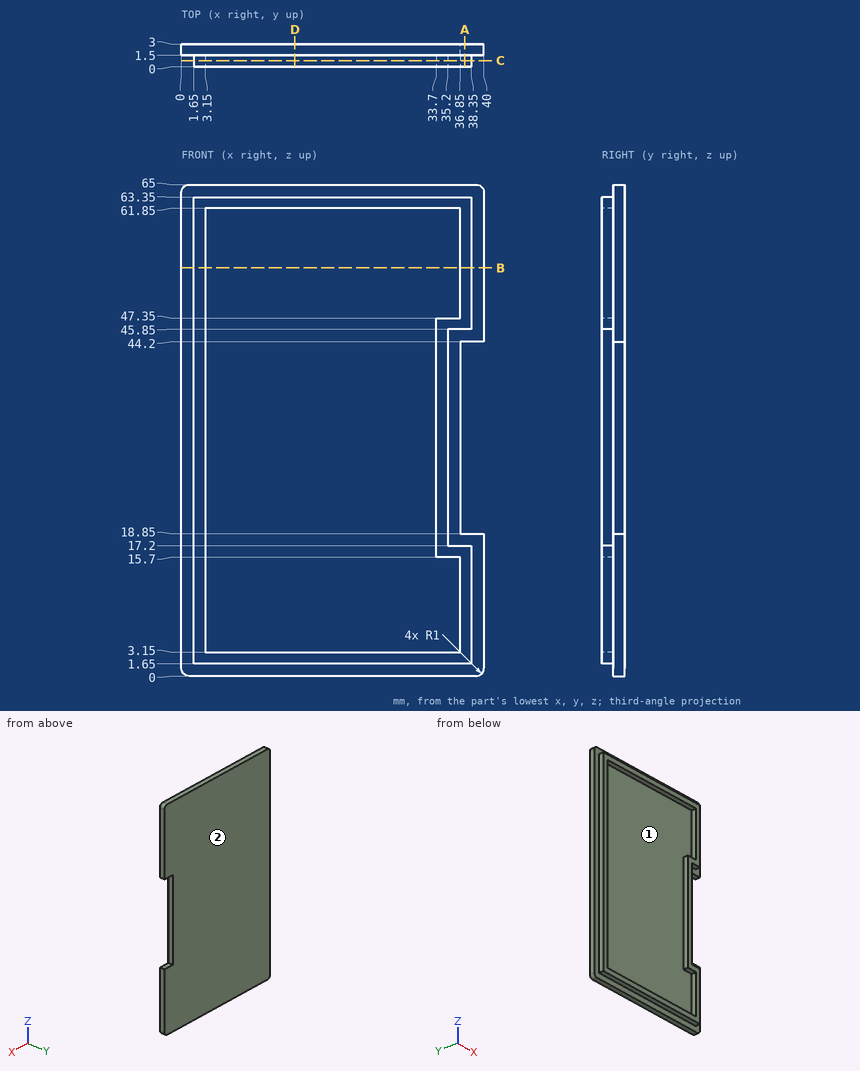
The drawing under review shows one solid part. Ordinate dimensions are in mm from its lowest x, y, z. Round coordinates to 2 decimals unless told otherwise and drop trailing zeros. Write each loop counter-clockwise with the first axis right and the second up, starting at its lowest first coordinate (ties: lowest second). Pieces come first, ordered by that corner, then holes. Notation, with made-up numbers: (33, -22) - (72, -22) arc R20 cw to (72, -12) - close; hole circle Ø10 at (-30, 8). An arc over 180 degrees is marked (long way). Put each result on its own line as item: value.
Q1. We need section D-D (x = 15). Give the boundary of the cut face in (y, z), and give its area (3 significant figures).
Solved:
outline: (0, 1.65) - (1.5, 1.65) - (1.5, 0) - (3, 0) - (3, 65) - (1.5, 65) - (1.5, 63.35) - (0, 63.35) - (0, 61.85) - (1.5, 61.85) - (1.5, 3.15) - (0, 3.15) - close
area: 102 mm2
Q2. We need section B-B (z = 54). Give the boundary of the cut face in (x, y).
Solved:
outline: (0, 1.5) - (1.65, 1.5) - (1.65, 0) - (3.15, 0) - (3.15, 1.5) - (36.85, 1.5) - (36.85, 0) - (38.35, 0) - (38.35, 1.5) - (40, 1.5) - (40, 3) - (0, 3) - close
Q3. Insertion check: pin 1 Ø5 at (x, z) = (30.5, 19) entering from -Y; pin 2 Ø1 at (y, z) = (2.5, 19.5) entering from +X; pin 3 Ø0.8 at (y, z) = (1, 11) entering from -X. Each pin has a flat end and moves straight along its axis. Give the tip position at first contact, or say it passes through.
Solved:
pin 1: stops at y = 1.5
pin 2: stops at x = 36.85
pin 3: stops at x = 1.65
Q4. Mouldability with a two-part tool opening along X and no side actions: class the marked faces 1 and 2 as released by +X, released by -X, zero draft, split by the parting line, or undercut.
Solved:
face 1: undercut
face 2: zero draft
Q5. We need section A-A (x = 37.5). Give the boundary of the cut face in (y, z), and give its area (3 significant figures).
Solved:
outline: (0, 1.65) - (1.5, 1.65) - (1.5, 0) - (3, 0) - (3, 18.85) - (1.5, 18.85) - (1.5, 17.2) - (0, 17.2) - close; (0, 45.85) - (1.5, 45.85) - (1.5, 44.2) - (3, 44.2) - (3, 65) - (1.5, 65) - (1.5, 63.35) - (0, 63.35) - close
area: 109 mm2
Q6. We need section C-C (y = 0.8). Give the boundary of the cut face in (x, z), and give its area (3 significant figures).
Solved:
outline: (1.65, 1.65) - (38.35, 1.65) - (38.35, 17.2) - (35.2, 17.2) - (35.2, 45.85) - (38.35, 45.85) - (38.35, 63.35) - (1.65, 63.35) - close; hole (3.15, 3.15) - (36.85, 3.15) - (36.85, 15.7) - (33.7, 15.7) - (33.7, 47.35) - (36.85, 47.35) - (36.85, 61.85) - (3.15, 61.85) - close
area: 296 mm2
Q7. Wall thickness on probe 1 along Z at (x, y) = (19, 1); probe 2 along Z at (x, y) = (2, 0.3); probe 3 along X at (y, z) = (1, 15.5): over which ranges is each line inside the solid? List them lowest first.
Solved:
probe 1: z = 1.65 to 3.15, 61.85 to 63.35
probe 2: z = 1.65 to 63.35
probe 3: x = 1.65 to 3.15, 36.85 to 38.35
